CAD build for the part. Positions are in the model's coordinates, mm. A direction names the side the tool comes from. Round coordinates to 2 decimals unless told otherwise and drop trailing zeros. Order: outer loops, then holes, each group sorted by start corner. A loop starts at its lowest first (then second) coordinate and runs counter-clockwise, first axis right, second up. Notation, with made-up numbers: M 57.5,84 L 115.5,84 A18 ccw 115.5,108 Z; hole C -1,-3 d4. An arc over 180 degrees is marked long. Put each result on its own line as item: value.
```python
from build123d import *

# Parameters (mm, degrees)
PAD_DEPTH   = 3
FILLET_R    = 1
FILLET001_R = 2.5


with BuildPart() as part:
    # Sketch → Pad (new body)
    with BuildSketch(Plane.XY):
        Polygon((25.598985, 32.987703), (25.598985, -7.012297), (22.348985, -7.012297), (22.348985, -10.012297), (12.448985, -10.012297), (12.448985, -7.012297), (9.198985, -7.012297), (9.198985, 32.987701), (12.448985, 32.987701), (12.448985, 35.987703), (22.348985, 35.987703), (22.348985, 32.987703), align=None)
    extrude(amount=PAD_DEPTH)

    # Fillet
    fillet_edges = [part.edges().sort_by_distance(p)[0] for p in [
        (22.348985, -10.012297, 1.5),
        (12.448985, -10.012297, 1.5),
        (22.348985, 35.987703, 1.5),
        (12.448985, 35.987703, 1.5),
    ]]
    fillet(fillet_edges, radius=FILLET_R)

    # Fillet001
    fillet001_edges = [part.edges().sort_by_distance(p)[0] for p in [
        (25.598985, -7.012297, 1.5),
        (25.598985, 32.987703, 1.5),
        (9.198985, -7.012297, 1.5),
        (9.198985, 32.987701, 1.5),
    ]]
    fillet(fillet001_edges, radius=FILLET001_R)


with BuildPart() as part_1:
    # Fillet001 placement: moved
    add(part.part.moved(Location((200, 100, 0))))


solid = part_1.part
```
Item 1: Tool access for faces 1 (the flat face through (222.349, 92, 1)), 2 (the flat face through (212.449, 134, 1)), 3 (the flat face through (222.349, 134, 1)): list every direction of +Z, -Z, +X, -X, +Y, -Y with a clear straight run to the whole face (end or side of a thin tool).
Answers below:
face 1: +Z, -Z, +X, -Y
face 2: +Z, -Z, -X, +Y
face 3: +Z, -Z, +X, +Y
Item 2: Band-saw the part on A-A on z = 2.15. Give the cut face in (x, y).
Answers below:
outline: M 209.2,95.49 A2.5 ccw 211.7,92.99 L 212.45,92.99 L 212.45,90.99 A1 ccw 213.45,89.99 L 221.35,89.99 A1 ccw 222.35,90.99 L 222.35,92.99 L 223.1,92.99 A2.5 ccw 225.6,95.49 L 225.6,130.49 A2.5 ccw 223.1,132.99 L 222.35,132.99 L 222.35,134.99 A1 ccw 221.35,135.99 L 213.45,135.99 A1 ccw 212.45,134.99 L 212.45,132.99 L 211.7,132.99 A2.5 ccw 209.2,130.49 Z
Item 3: Probe line 1 along Y through (x, z) = (212.25, 2.25); line 2 along Y through (x, z) = (210, 0.85); line 3 along X through (y, z) = (94.5, 2.55). List the from-to ranges inside material, lowest first. Write a range as [from, to].
Answers below:
line 1: [92.99, 132.99]
line 2: [93.65, 132.32]
line 3: [209.4, 225.4]
Item 4: Band-saw the part on B-B on y = 133.5. Give the cut face in (x, z), and give its area (3 significant figures).
Answers below:
outline: M 212.45,0 L 222.35,0 L 222.35,3 L 212.45,3 Z
area: 29.7 mm²
Item 5: Pin check, flat tips, straight feed: P1, Ø0.6, axis at y = 133.5, z = 1, coming from the +X side; P2, Ø0.8, axis at x = 212, z = 1.5, coming from the -Y side; P3, Ø1.6, axis at y = 91.5, z = 1.5, coming from the -X side. Stop position of each tip, or through.
Answers below:
P1: x = 222.35
P2: y = 92.99
P3: x = 212.45
